Input: part model. Units: mm. Frame: model coordinates. A direction names the side the tool comes from. Coordinates: 2 decimals unless noted, no trailing zeros. Write each loop counter-clockwise with the first axis right and the second up, starting at its lowest first coordinate (ties: lowest second). Pieces come first, ordered by that corner, then holes. Notation, with made-up numbers: (35.5, 86) - (86.5, 86) arc R18 cw to (86.5, 114) - close; hole circle Ø7 at (74.5, -9). An arc over 180 degrees is marked (long way). Use a Markdown table: item, result. Add a question column.
Q1. Pin query (flat end, axial travel): P1, Ø1, axis at x = -3, z = -3, coming from the -Y side; P2, Ø4, axis at x = -36, z = 0, coming from the +Y side; P3, Ø3, axis at y = 8.5, z = 4, coming from the +X side. Return the tip coordinate at first contact, or that it passes through.
Q2. Set-up query: faces 1 (the face through (30, 9, 0)), 2 (the face through (26, 5, 0)), 3 (the face through (33, 0, 0)), 4 (the face through (-36, 4, 2)). Return all of +Z, -Z, +X, -X, +Y, -Y with unobstructed straight access to the full face (end or side cutting, diameter ignored); none if empty.
Q3. Section query A-A (y = 8). Return the cut outline in (x, z), then the cut area to 3 significant figures.
Q4. Section query C-C (z = 0). Return the cut outline in (x, y).
Q5. Section query B-B (y = 2). Return the cut outline in (x, z).
Q6. Material intervals for probe 1 along Z at (x, y) = (36, 1.4); probe 2 along X at (y, z) = (2.75, 0.5); probe 3 along X at (y, z) = (1.25, -4.5), sorted ascending. Write a range as from..to.
Q7. Mould query, pull axis X, two halves, no side actions, for faces 5 (the face through (1, 12, -10)), 6 (the face through (42.5, 2, 0)), 7 (the face through (0, 10, 0)). Classes: released by +X, released by -X, zero draft, split by the parting line, or undercut.
Q8. Section query D-D (x = 36). Return the cut outline in (y, z), then the cut area to 3 significant figures.
Autodesk Inventor part; units mm, degrees
ref_plane "YZ Plane" through (0, 0, 0) normal (1, 0, 0) x (0, 1, 0)
ref_plane "XZ Plane" through (0, 0, 0) normal (0, 1, 0) x (-1, 0, 0)
ref_plane "XY Plane" through (0, 0, 0) normal (0, 0, 1) x (1, 0, 0)
sketch "Sketch1" plane through (0, 0, 0) normal (0, 1, 0) x (-1, 0, 0)
  line L0 (-42.5, -10) -> (42.5, -10)
  line L1 (42.5, -10) -> (42.5, 10)
  line L2 (42.5, 10) -> (-42.5, 10)
  line L3 (-42.5, 10) -> (-42.5, -10)
  line L4 (-42.5, -10) -> (42.5, 10) construction
  line L5 (42.5, -10) -> (-42.5, 10) construction
  line L6 (-30, -10) -> (30, -10)
  line L7 (30, -10) -> (30, 10)
  line L8 (30, 10) -> (-30, 10)
  line L9 (-30, 10) -> (-30, -10)
  line L10 (-30, -10) -> (30, 10) construction
  line L11 (30, -10) -> (-30, 10) construction
  circle A0 centre (36, 0) radius 1.75
  circle A1 centre (-36, 0) radius 1.75
  line L12 (0, 10) -> (0, -10) construction
  line L13 (30, 10) -> (26, 10)
  line L14 (26, 10) -> (26, -10)
  line L15 (26, -10) -> (30, -10)
  line L16 (30, -10) -> (30, 10)
  line L17 (-30, -10) -> (-26, -10)
  line L18 (-26, -10) -> (-26, 10)
  line L19 (-26, 10) -> (-30, 10)
  line L20 (-30, 10) -> (-30, -10)
  point P0 (0, 0)
  point P1 (0, 0)
  dimension "d0" = 72
  dimension "d1" = 60
  dimension "d2" = 85
  dimension "d3" = 3.5
  dimension "d4" = 20
  dimension "d7" = 4
extrude "Extrusion1" add sketch "Sketch1" along normal blind 4 contours L3 L2 L9 L0 | L7 L2 L1 L0
extrude "Extrusion2" add sketch "Sketch1" along normal blind 10 contours L9 L2 L18 L0 | L14 L2 L7 L0
extrude "Extrusion3" add sketch "Sketch1" along normal blind 4 from surface at 10 contours L9 L2 L18 L0 | L18 L2 L14 L0 | L14 L2 L7 L0
properties part number "cable_protector"
Values follow:
| question | item | result |
|---|---|---|
| 1 | P1 | y = 10 |
| 1 | P2 | y = 4 |
| 1 | P3 | x = 30 |
| 2 | face 1 | +Z, -Z, +X, +Y |
| 2 | face 2 | +Z, -Z, -Y |
| 2 | face 3 | +Z, -Z, +X, -X, -Y |
| 2 | face 4 | +Z, -Z, -X, +Y |
| 3 | outline | (-30, -10) - (-26, -10) - (-26, 10) - (-30, 10) - close; (26, -10) - (30, -10) - (30, 10) - (26, 10) - close |
| 3 | area | 160 mm2 |
| 4 | outline | (-42.5, 0) - (-37.75, 0) - (-37.75, 4) - (-42.5, 4) - close; (-34.25, 0) - (-26, 0) - (-26, 10) - (26, 10) - (26, 0) - (34.25, 0) - (34.25, 4) - (30, 4) - (30, 14) - (-30, 14) - (-30, 4) - (-34.25, 4) - close; (37.75, 0) - (42.5, 0) - (42.5, 4) - (37.75, 4) - close |
| 5 | outline | (-42.5, -10) - (-26, -10) - (-26, 10) - (-42.5, 10) - close; (26, -10) - (42.5, -10) - (42.5, 10) - (26, 10) - close; hole circle Ø3.5 at (-36, 0); hole circle Ø3.5 at (36, 0) |
| 6 | probe 1 | -10..-1.75, 1.75..10 |
| 6 | probe 2 | -42.5..-37.68, -34.32..-26, 26..34.32, 37.68..42.5 |
| 6 | probe 3 | -42.5..-26, 26..42.5 |
| 7 | face 5 | zero draft |
| 7 | face 6 | released by +X |
| 7 | face 7 | undercut |
| 8 | outline | (0, -10) - (4, -10) - (4, -1.75) - (0, -1.75) - close; (0, 1.75) - (4, 1.75) - (4, 10) - (0, 10) - close |
| 8 | area | 66.0 mm2 |
